from build123d import *

# Parameters (mm, degrees)
F0_R     = 24.385
F1_DEPTH = 30
F2_R     = 22
F3_DEPTH = 8
F4_R     = 3
F6_DEPTH = 20
F7_R     = 1


with BuildPart() as f1:
    # F0 (on Top) → F1 (new body)
    with BuildSketch(Plane.XY):
        Circle(F0_R)
    extrude(amount=F1_DEPTH)

    # F2 (on face) → F3 (cut)
    with BuildSketch(Plane.XY.offset(30)):
        Circle(F2_R)
    extrude(amount=-F3_DEPTH, mode=Mode.SUBTRACT)

    # F4
    f4_edges = [f1.edges().sort_by_distance(p)[0] for p in [
        (-22, 0, 22),
    ]]
    fillet(f4_edges, radius=F4_R)

    # F5 (on face) → F6 (cut)
    with BuildSketch(Plane.XY.offset(22)):
        with BuildLine():
            Line((-1.2082039889, -0.5004544783), (-18.9934079437, -0.5004544783))
            ThreePointArc((-18.9934079437, -0.5004544783), (-17.5537111177, -7.2709852149), (-13.7842423101, -13.0764927995))
            Line((-13.7842423101, -13.0764927995), (-1.2082039889, -0.5004544783))
        make_face()
        with BuildLine():
            ThreePointArc((-13.7842423101, 13.0764927995), (-17.5537111177, 7.2709852149), (-18.9934079437, 0.5004544783))
            Line((-18.9934079437, 0.5004544783), (-1.2082039889, 0.5004544783))
            Line((-1.2082039889, 0.5004544783), (-13.7842423101, 13.0764927995))
        make_face()
        with BuildLine():
            Line((-0.5004544783, -1.2082039889), (-13.0764927995, -13.7842423101))
            ThreePointArc((-13.0764927995, -13.7842423101), (-7.2709852149, -17.5537111177), (-0.5004544783, -18.9934079437))
            Line((-0.5004544783, -18.9934079437), (-0.5004544783, -1.2082039889))
        make_face()
        with BuildLine():
            Line((0.5004544783, -1.2082039889), (0.5004544783, -18.9934079437))
            ThreePointArc((0.5004544783, -18.9934079437), (7.2709852149, -17.5537111177), (13.0764927995, -13.7842423101))
            Line((13.0764927995, -13.7842423101), (0.5004544783, -1.2082039889))
        make_face()
        with BuildLine():
            Line((1.2082039889, -0.5004544783), (13.7842423101, -13.0764927995))
            ThreePointArc((13.7842423101, -13.0764927995), (17.5537111177, -7.2709852149), (18.9934079437, -0.5004544783))
            Line((18.9934079437, -0.5004544783), (1.2082039889, -0.5004544783))
        make_face()
        with BuildLine():
            Line((1.2082039889, 0.5004544783), (18.9934079437, 0.5004544783))
            ThreePointArc((18.9934079437, 0.5004544783), (17.5537111177, 7.2709852149), (13.7842423101, 13.0764927995))
            Line((13.7842423101, 13.0764927995), (1.2082039889, 0.5004544783))
        make_face()
        with BuildLine():
            Line((0.5004544783, 1.2082039889), (13.0764927995, 13.7842423101))
            ThreePointArc((13.0764927995, 13.7842423101), (7.2709852149, 17.5537111177), (0.5004544783, 18.9934079437))
            Line((0.5004544783, 18.9934079437), (0.5004544783, 1.2082039889))
        make_face()
        with BuildLine():
            Line((-0.5004544783, 1.2082039889), (-0.5004544783, 18.9934079437))
            ThreePointArc((-0.5004544783, 18.9934079437), (-7.2709852149, 17.5537111177), (-13.0764927995, 13.7842423101))
            Line((-13.0764927995, 13.7842423101), (-0.5004544783, 1.2082039889))
        make_face()
    extrude(amount=-F6_DEPTH, mode=Mode.SUBTRACT)

    # F7
    f7_edges = [f1.edges().sort_by_distance(p)[0] for p in [
        (-18.993408, 0.500454, 12),
        (-18.993408, -0.500454, 12),
        (-13.076493, 13.784242, 12),
        (-13.784242, 13.076493, 12),
        (0.500454, 18.993408, 12),
        (-0.500454, 18.993408, 12),
        (13.076493, 13.784242, 12),
        (13.784242, 13.076493, 12),
        (18.993408, 0.500454, 12),
        (18.993408, -0.500454, 12),
        (13.076493, -13.784242, 12),
        (13.784242, -13.076493, 12),
        (0.500454, -18.993408, 12),
        (-0.500454, -18.993408, 12),
        (-13.076493, -13.784242, 12),
        (-13.784242, -13.076493, 12),
        (-0.500454, -1.208204, 12),
        (-1.208204, -0.500454, 12),
        (-1.208204, 0.500454, 12),
        (-0.500454, 1.208204, 12),
        (0.500454, 1.208204, 12),
        (1.208204, 0.500454, 12),
        (1.208204, -0.500454, 12),
        (0.500454, -1.208204, 12),
    ]]
    fillet(f7_edges, radius=F7_R)


solid = f1.part
Could you check a few things on this model? Use its own coordinates, in mm. Round coordinates to 2 decimals unless told otherwise and drop trailing zeros. Use a Markdown table: item, result.
1. We'd pull the mould along Y, two halves only. Please class faces 1 (the face through (-19.35, -14.84, 14.79)), 2 (the face through (-4, 22, 30)), 3 (the face through (7.195, -17.585, 12.14)): +Y half, -Y half, draft (parallel to the pull), parting line (faces both ways), or undercut.
Answer key:
| item | result |
|---|---|
| face 1 | parting line |
| face 2 | draft |
| face 3 | undercut |
2. For pin 1 Ø1.5 at (x, z) = (14.5, 4) entering from +Y; pin 2 Ø3.5 at (x, y) = (7, -9) entering from +Z; pin 3 Ø1 at (x, y) = (13, 14) entering from -Z; pin 4 Ø11.5 at (y, z) = (8.5, 14) entering from -X, each with a flat end and sliding along its axis, tell me the tip position at first contact or that it passes through.
Answer key:
| item | result |
|---|---|
| pin 1 | stops at y = 20.14 |
| pin 2 | stops at z = 22 |
| pin 3 | stops at z = 0 |
| pin 4 | stops at x = -24.23 |
3. If we section it at A-A (z = 11): State how many separate pieces and enclosed holes the cut face has, then the cut area to 3 significant figures.
Answer key:
| item | result |
|---|---|
| separate pieces | 1 |
| enclosed holes | 8 |
| area | 895 mm^2 |
4. Please list where these lines run through material, in increasing order: probe 1 along Y at (x, z) = (0, 29) (3 decimals); probe 2 along Y at (x, z) = (10, 20); probe 3 along X at (y, z) = (-8, 5).
Answer key:
| item | result |
|---|---|
| probe 1 | y = -24.385 to -22, 22 to 24.385 |
| probe 2 | y = -22.24 to -16.16, -10.71 to -9.29, -0.5 to 0.5, 9.29 to 10.71, 16.16 to 22.24 |
| probe 3 | x = -23.04 to -17.23, -8.71 to -7.29, -0.5 to 0.5, 7.29 to 8.71, 17.23 to 23.04 |
